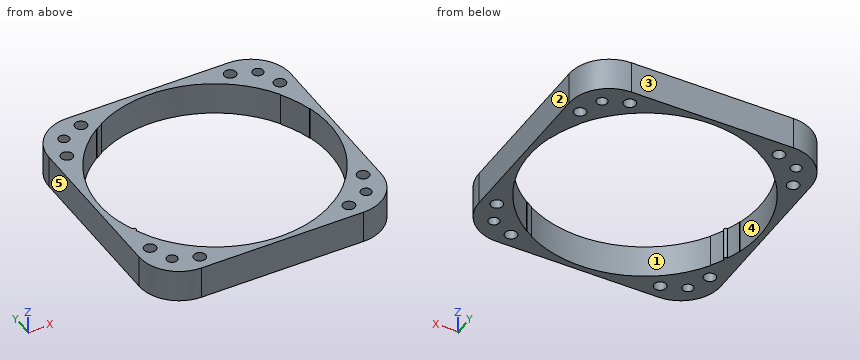
Autodesk Inventor part; units mm, degrees
ref_plane "YZ Plane" through (0, 0, 0) normal (1, 0, 0) x (0, 1, 0)
ref_plane "XZ Plane" through (0, 0, 0) normal (0, 1, 0) x (-1, 0, 0)
ref_plane "XY Plane" through (0, 0, 0) normal (0, 0, 1) x (1, 0, 0)
sketch "Sketch1" plane through (0, 0, 0) normal (0, 0, 1) x (1, 0, 0)
  circle A0 centre (0, 0) radius 57.5
  circle A1 centre (0, 0) radius 60.5
  line L0 (-40.5, 60.5) -> (40.5, 60.5)
  line L1 (60.5, 40.5) -> (60.5, -40.5)
  line L2 (40.5, -60.5) -> (-40.5, -60.5)
  line L3 (-60.5, -40.5) -> (-60.5, 40.5)
  arc A2 (-40.5, 60.5) -> (-60.5, 40.5) centre (-40.5, 40.5) ccw
  arc A3 (60.5, 40.5) -> (40.5, 60.5) centre (40.5, 40.5) ccw
  arc A4 (40.5, -60.5) -> (60.5, -40.5) centre (40.5, -40.5) ccw
  arc A5 (-60.5, -40.5) -> (-40.5, -60.5) centre (-40.5, -40.5) ccw
  dimension "d0" = 115
  dimension "d1" = 121
  dimension "d2" = 20
extrude "Extrusion1" add sketch "Sketch1" along normal blind 16.25
sketch "Sketch3" plane through (0, 0, 16.25) normal (0, 0, 1) x (1, 0, 0)
  circle A0 centre (-48.5, -48.5) radius 2.65
  circle A1 centre (-53.2449, -37.2825) radius 2.15
  circle A2 centre (-37.2825, -53.2449) radius 2.15
  circle A3 centre (37.2825, -53.2449) radius 2.15
  circle A4 centre (48.5, -48.5) radius 2.65
  circle A5 centre (53.2449, -37.2825) radius 2.15
  circle A6 centre (53.2449, 37.2825) radius 2.15
  circle A7 centre (48.5, 48.5) radius 2.65
  circle A8 centre (37.2825, 53.2449) radius 2.15
  circle A9 centre (-37.2825, 53.2449) radius 2.15
  circle A10 centre (-48.5, 48.5) radius 2.65
  circle A11 centre (-53.2449, 37.2825) radius 2.15
  point P0 (0, 0)
extrude "Extrusion3" cut sketch "Sketch3" against normal through all
sketch "Sketch4" plane through (0, 0, 16.25) normal (0, 0, 1) x (1, 0, 0)
  circle A0 centre (-37.2825, -53.2449) radius 2.15
  circle A1 centre (-37.2825, -53.2449) radius 3
  circle A2 centre (-53.2449, -37.2825) radius 2.15
  circle A3 centre (-53.2449, -37.2825) radius 3
  circle A4 centre (-53.2449, 37.2825) radius 2.15
  circle A5 centre (-53.2449, 37.2825) radius 3
  circle A6 centre (-37.2825, 53.2449) radius 2.15
  circle A7 centre (-37.2825, 53.2449) radius 3
  circle A8 centre (37.2825, 53.2449) radius 2.15
  circle A9 centre (37.2825, 53.2449) radius 3
  circle A10 centre (53.2449, 37.2825) radius 2.15
  circle A11 centre (53.2449, 37.2825) radius 3
  circle A12 centre (53.2449, -37.2825) radius 2.15
  circle A13 centre (53.2449, -37.2825) radius 3
  circle A14 centre (37.2825, -53.2449) radius 2.15
  circle A15 centre (37.2825, -53.2449) radius 3
  point P0 (0, 0)
  point P1 (48.5, -48.5)
  dimension "d28" = 6
  dimension "d29" = 6
  dimension "d30" = 6
  dimension "d31" = 6
  dimension "d32" = 6
  dimension "d33" = 6
  dimension "d34" = 6
  dimension "d36" = 6
extrude "Extrusion4" cut sketch "Sketch4" against normal through all contours A0 | A1 | A2 | A3 | A4 | A5 | A6 | A7 | A8 | A9 | A10 | A11 | A12 | A13 | A14 | A15
sketch "Sketch5" plane through (0, 0, 16.25) normal (0, 0, 1) x (1, 0, 0)
  arc A0 (-51.9873, -22.1262) -> (-53.291, -21.5943) centre (-52.9074, -22.5178) ccw
  arc A1 (-52.5078, -23.4345) -> (-51.9873, -22.1262) centre (-52.9074, -22.5178) ccw
  circle A2 centre (0, 0) radius 57.55
  circle A3 centre (-52.9074, -22.5178) radius 0.95
  circle A4 centre (0, 0) radius 57.75
  line L0 (55.7822, 14.9468) -> (-70.3053, -18.8382)
  line L1 (40.5, 60.5) -> (-40.5, 60.5)
  line L2 (49.5014, 29.7434) -> (-78.6926, -47.2833)
  line L3 (32.5757, -47.6853) -> (-33.549, 49.11)
  line L4 (29.1077, -49.8779) -> (-30.5513, 52.3515)
  point P0 (-55.7822, -14.9468)
  point P1 (-55.589, -14.895)
  point P2 (-53.3179, -21.6611)
  point P3 (-52.5746, -23.4076)
  point P4 (-49.33, -29.6404)
  point P5 (-49.5014, -29.7434)
  point P6 (29.0069, -49.7051)
  point P7 (32.4629, -47.5201)
  point P8 (-29.1077, 49.8779)
  point P9 (-29.0069, 49.7051)
  point P10 (-32.4629, 47.5201)
  point P11 (-32.5757, 47.6853)
  dimension "d39" = 115.1
  dimension "d40" = 115.5
  dimension "d41" = 15
  dimension "d42" = 16
extrude "Extrusion5" cut sketch "Sketch5" against normal through all contours A2 L3 L0 | A2 L0 A4 L3 | A2 L4 L3 | L2 L4 A2 | A2 L4 A4 L2 | L2 A2 A3 L0 | L4 A2 L2 | L0 A2 L3 | L3 A2 L4 | L4 A4 L2 A2 | L0 A4 L3 A2
sketch "Sketch6" plane through (0, 0, 16.25) normal (0, 0, 1) x (1, 0, 0)
  arc A0 (-52.5078, -23.4345) -> (-51.9873, -22.1262) centre (-52.9074, -22.5178) ccw
  arc A1 (-51.9873, -22.1262) -> (-53.291, -21.5943) centre (-52.9074, -22.5178) ccw
  arc A2 (-53.2722, -21.6407) -> (-52.5282, -23.3888) centre (0, 0) ccw
  circle A3 centre (-52.9074, -22.5178) radius 0.95
  point P0 (-52.5282, -23.3888)
extrude "Extrusion6" add sketch "Sketch6" against normal up to surface (16.25 mm away) contours A3 A2 picked at (-52.6277, -22.3682)
equation "\"d28\" = d31"
equation "\"d29\" = d31"
equation "\"d30\" = d31"
equation "\"d32\" = d31"
equation "\"d33\" = d31"
equation "\"d34\" = d31"
equation "\"d36\" = d31"
properties part number "stator_center_00_p" material "PC/ABS Plastic"
Check sheet for the modelled part. Datum: model origin and axes. Units: mm. Face numbers are marked on the shaded views. A direction names the side the tool comes from. Give positions to 0.01 mm unless a question says otherwise; leave off trailing zeros. Write each loop counter-clockwise with the first axis right and the second up, starting at its lowest first coordinate (ties: lowest second). Pieces come first, ordered by that corner, then holes. Notation, with made-up numbers: (-27, 53) -> (-8, 53) arc R19 cw to (-8, 71) -> close; hole circle Ø11 at (86, -39). An arc over 180 degrees is marked (long way). Use CSV: the item, a comma, the result in double quotes. Start each with the question number.
Q1. Scan lines: line 1 along X through (y, z) = (1, 5.5); line 2 along X through (y, z) = (-46.5, 3.5); line 3 along Y through (x, z) = (1.5, 13). Record each from-to range of solid material in increasing order.
Q2. Depth check by flat-ended pin: P1, Ø5, axis at x = -53.24, y = 37.28, coming from the +Z side; P2, Ø5, axis at x = -44.5, z = 3, coming from the -Y side. Enter the tip coordinate at first touch or a pass-through.
Q3. Tool access check on the marked faces 4 and 5. Record the directions out of +Z, -Z, +X, -X, +Y, -Y that give a thin tool (end or side, any length) a straight path to the whole face; none if there is none.
Q4. Release check for a two-part mould opening along X. For the marked faces 1, 2 and 3 record: +X half, -X half, draft (parallel to the pull), parting line (faces both ways), or undercut.
Q5. Cross-section at A-A on x = -38. Enter the section's corners in (y, z).
Q6. Cross-section at C-C on z = 9.25. Count the separate pieces of the cut face and the enclosed holes in it, and give its area (3 significant figures).
Q7. Cross-section at B-B on y = 7. Enter the section's corners in (x, z), and give its area (3 significant figures).
Q8. Cross-section at D-D on y = -42. Enter the section's corners in (x, z).
Working result:
1,line 1,"x = -60.5 to -57.74, 57.74 to 60.5"
1,line 2,"x = -59.58 to -50.24, -46.76 to -34.25, 34.25 to 46.76, 50.24 to 59.58"
1,line 3,"y = -60.5 to -57.73, 57.73 to 60.5"
2,P1,"passes through"
2,P2,"stops at y = -60.44"
3,face 4,"+Z, -Z"
3,face 5,"+Z, -Z, -X, +Y, -Y"
4,face 1,"undercut"
4,face 2,"+X half"
4,face 3,"draft"
5,outline,"(-60.5, 0) -> (-56.16, 0) -> (-56.16, 16.25) -> (-60.5, 16.25) -> close; (-50.33, 0) -> (-43.49, 0) -> (-43.49, 16.25) -> (-50.33, 16.25) -> close; (43.49, 0) -> (50.33, 0) -> (50.33, 16.25) -> (43.49, 16.25) -> close; (56.16, 0) -> (60.5, 0) -> (60.5, 16.25) -> (56.16, 16.25) -> close"
6,separate pieces,"1"
6,enclosed holes,"13"
6,area,"3,520 mm^2"
7,outline,"(-60.5, 0) -> (-57.32, 0) -> (-57.32, 16.25) -> (-60.5, 16.25) -> close; (57.32, 0) -> (60.5, 0) -> (60.5, 16.25) -> (57.32, 16.25) -> close"
7,area,"103 mm^2"
8,outline,"(-60.44, 0) -> (-39.64, 0) -> (-39.64, 16.25) -> (-60.44, 16.25) -> close; (39.64, 0) -> (60.44, 0) -> (60.44, 16.25) -> (39.64, 16.25) -> close"
